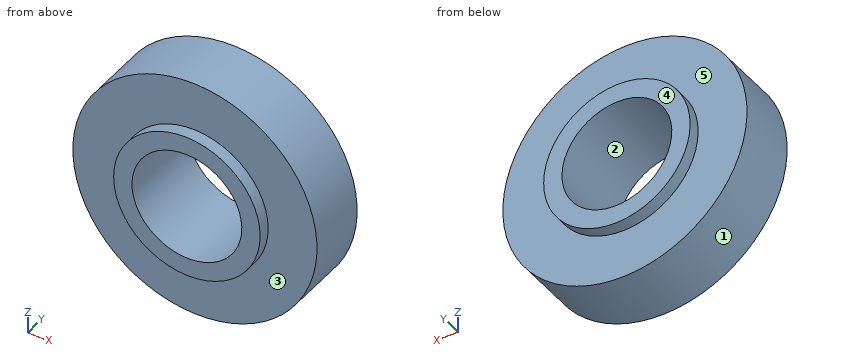
```python
from build123d import *

# Parameters (mm, degrees)
SKETCH1_R           = 10
SKETCH1_R_2         = 4.5
BOSS_EXTRUDE1_DEPTH = 3.5
SKETCH2_R           = 13
SKETCH2_R_2         = 6
CUT_EXTRUDE1_DEPTH  = 1


with BuildPart() as part:
    # Sketch1 → Boss-Extrude1 (new, symmetric)
    with BuildSketch(Plane(origin=(0, 0, 0), x_dir=(1, 0, 0), z_dir=(0, 1, 0))):
        with Locations(Location((0, 0, 0), (0, 0, 270))):
            Circle(SKETCH1_R)
        with Locations(Location((0, 0, 0), (0, 0, 270))):
            Circle(SKETCH1_R_2, mode=Mode.SUBTRACT)
    extrude(amount=BOSS_EXTRUDE1_DEPTH, both=True)

    # Sketch2 → Cut-Extrude1 (cut)
    with BuildSketch(Plane(origin=(0, 3.5, 0), x_dir=(1, 0, 0), z_dir=(0, 1, 0))):
        Circle(SKETCH2_R)
        with Locations(Location((0, 0, 0), (0, 0, 270))):
            Circle(SKETCH2_R_2, mode=Mode.SUBTRACT)
    cut_extrude1 = extrude(amount=-CUT_EXTRUDE1_DEPTH, mode=Mode.SUBTRACT)

    # Mirror1: Cut-Extrude1 across plane
    add(cut_extrude1.mirror(Plane.ZX), mode=Mode.SUBTRACT)


solid = part.part
```
For this review, take the finished solid that the model builds, in its own axes (mm). Face numbers are marked on the shaded views. A direction names the side the tool comes from. Round coordinates to 2 decimals unless told otherwise and drop trailing zeros. Write each loop counter-clockwise with the first axis right and the second up, starting at its lowest first coordinate (ties: lowest second). Pieces come first, ordered by that corner, then holes. Notation, with made-up numbers: (-30.5, -8) - (-16.5, -8) arc R10 ccw to (-16.5, 11) - close; hole circle Ø4 at (88.25, 61). An arc over 180 degrees is marked (long way). Use CSV: the item, a comma, the result in double quotes.
1) Wall thickness on line 1 along X through (y, z) = (-1, 0); line 2 along Y through (x, z) = (4.5, -8.25); line 3 along Z through (x, y) = (8, -0.5): over which ranges is each line inside the solid? List them lowest first. Write a range as from..to.
Conclusion:
line 1,"x = -10..-4.5, 4.5..10"
line 2,"y = -2.5..2.5"
line 3,"z = -6..6"
2) Add section A-A on z = 0. Write out the cut boundary in (x, y), and give its area (3 significant figures).
Conclusion:
outline,"(-10, -2.5) - (-6, -2.5) - (-6, -3.5) - (-4.5, -3.5) - (-4.5, 3.5) - (-6, 3.5) - (-6, 2.5) - (-10, 2.5) - close; (4.5, -3.5) - (6, -3.5) - (6, -2.5) - (10, -2.5) - (10, 2.5) - (6, 2.5) - (6, 3.5) - (4.5, 3.5) - close"
area,"61.0 mm^2"
3) Add section D-D on x = -5. Write out the cut boundary in (y, z), and give its area (3 significant figures).
Conclusion:
outline,"(-3.5, -3.32) - (-2.5, -3.32) - (-2.5, -8.66) - (2.5, -8.66) - (2.5, -3.32) - (3.5, -3.32) - (3.5, 3.32) - (2.5, 3.32) - (2.5, 8.66) - (-2.5, 8.66) - (-2.5, 3.32) - (-3.5, 3.32) - close"
area,"99.9 mm^2"
4) For the marked faces 4 and 5, list the 3-axis set-ups (+Z, -Z, +X, -X, +Y, -Y) from which the entire face can be reached by the end or side of a thin tool; tool diameter is ignored.
Conclusion:
face 4,"+Z, -Z, +X, -X, +Y"
face 5,"+Y"
5) Clearance check with flat-ended pins moving along their axes: pin 1 Ø1.5 at (x, y) = (-2, 1.5) entering from +Z; pin 2 Ø2 at (x, z) = (7, -5.5) entering from -Y; pin 3 Ø1.5 at (x, y) = (-4, -1.5) entering from -Z. State where each tip first meets the part, or that it passes through.
Conclusion:
pin 1,"stops at z = 9.92"
pin 2,"stops at y = -2.5"
pin 3,"stops at z = -9.46"
6) The part is to be moulded in two halves that separate along Z. For the marked faces 1, 2 and 3, say which applies: pulls with the +Z half, pulls with the -Z half, needs draft (parallel to the pull), parting line crosses it, or undercut.
Conclusion:
face 1,"parting line crosses it"
face 2,"undercut"
face 3,"needs draft"
7) Add section B-B on x = 0. Write out the cut boundary in (y, z).
Conclusion:
outline,"(-3.5, -6) - (-2.5, -6) - (-2.5, -10) - (2.5, -10) - (2.5, -6) - (3.5, -6) - (3.5, -4.5) - (-3.5, -4.5) - close; (-3.5, 4.5) - (3.5, 4.5) - (3.5, 6) - (2.5, 6) - (2.5, 10) - (-2.5, 10) - (-2.5, 6) - (-3.5, 6) - close"
8) Add section C-C on y = -1.25. Write out the cut boundary in (x, z).
Conclusion:
outline,"circle Ø20 at (0, 0); hole circle Ø9 at (0, 0)"
